Study the drawing (mm; zero at the part's minimum x, y, z) and answer. A direction names the side the tool comes from. Coordinates: 2 decimals unless noted, no trailing zeros. Order: outer loops, then holes, each group sorted by start corner. A loop starts at its lowest first (then second) coordinate and runs counter-clockwise, first axis right, second up. Notation, with made-up numbers: M 61.25,71.25 L 83.25,71.25 A25 ccw 83.25,102.25 Z; hole C 0,13 d10. An arc over 180 degrees is marked long. Put each result on its own line as item: value.
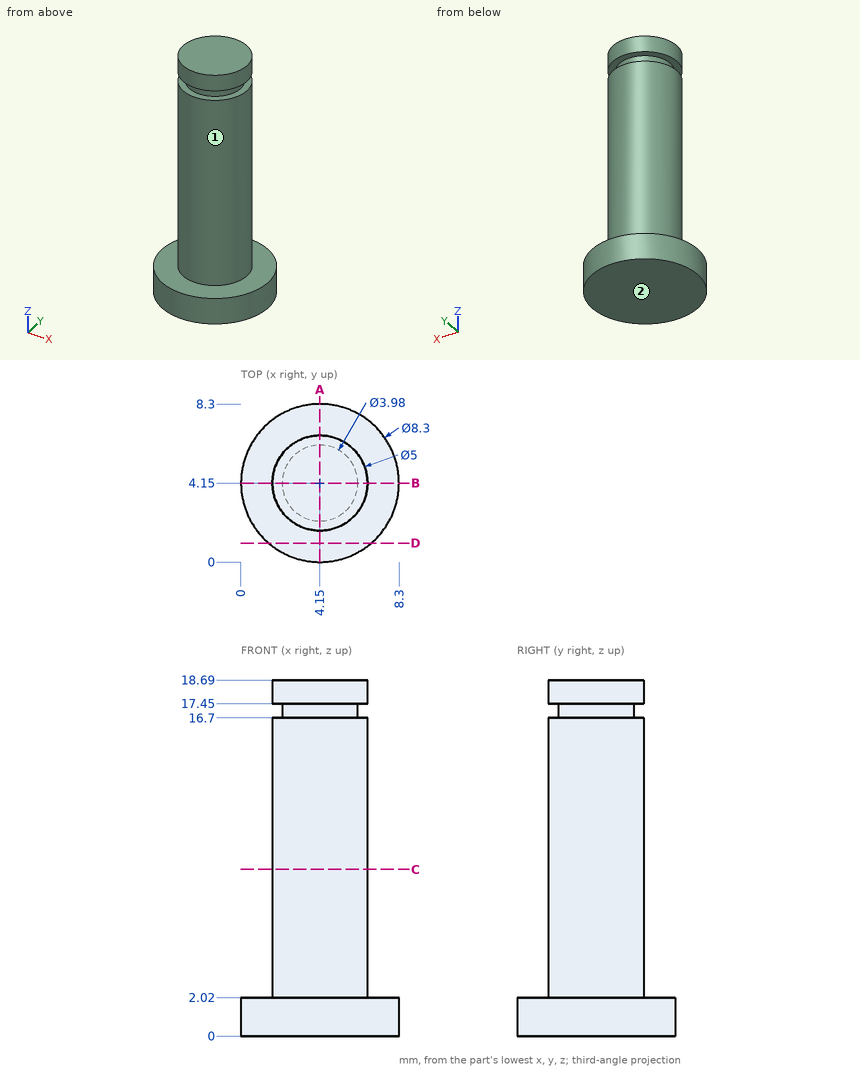
Q1. Given pin 1 (2 mm diameter, centred on x = 3.5, z = 13, fed in from +Y); pin 2 (1 mm diameter, centred on y = 2, z = 4.5, fed in from -X), each flat-ended and moving along its own axis, determine where each tip first touches the part or whether it passes through.
Answers below:
pin 1: stops at y = 6.65
pin 2: stops at x = 2.27
Q2. Find section A-A on x = 4.15. Write down the section's boundary in (y, z), plus the area to 3 significant figures.
Answers below:
outline: M 0,0 L 8.3,0 L 8.3,2.02 L 6.65,2.02 L 6.65,16.7 L 6.14,16.7 L 6.14,17.45 L 6.65,17.45 L 6.65,18.69 L 1.65,18.69 L 1.65,17.45 L 2.16,17.45 L 2.16,16.7 L 1.65,16.7 L 1.65,2.02 L 0,2.02 Z
area: 99.4 mm^2
Q3. A tool of negligible diameter and unlimited length cuts with its end or side. For the marked faces 1 and 2, from which of +Z, -Z, +X, -X, +Y, -Y can it reach the whole face along a straight path? Write none if from no direction.
Answers below:
face 1: +Z
face 2: -Z, +X, -X, +Y, -Y
Q4. Find section D-D on y = 1. Write down the section's boundary in (x, z), plus the area to 3 significant figures.
Answers below:
outline: M 1.45,0 L 6.85,0 L 6.85,2.02 L 1.45,2.02 Z
area: 10.9 mm^2
Q5. Consider line 1 along Z through (x, y) = (6.25, 3.5); line 2 along Z through (x, y) = (2.75, 1); line 3 along Y through (x, z) = (4.25, 3.25). Determine where each line is inside the solid, lowest interval first.
Answers below:
line 1: z = 0 to 16.7, 17.45 to 18.69
line 2: z = 0 to 2.02
line 3: y = 1.65 to 6.65
Q6. Find section C-C on z = 8.75. Write down the section's boundary in (x, y), plus the area to 3 significant figures.
Answers below:
outline: C 4.15,4.15 d5
area: 19.6 mm^2
